from build123d import *

# Parameters (mm, degrees)
SKETCH1_W           = 15
SKETCH1_H           = 28.0162
SKETCH1_R           = 0.889
BOSS_EXTRUDE1_DEPTH = 3.175
SKETCH1_3_W         = 15
SKETCH1_3_H         = 12.7
SKETCH1_3_R         = 3.1115
BOSS_EXTRUDE2_DEPTH = 12.7


with BuildPart() as part:
    # Sketch1 → Boss-Extrude1 (new body)
    with BuildSketch(Plane(origin=(0, 0, 0), x_dir=(1, 0, 0), z_dir=(0, 1, 0))):
        with Locations((7.5, -26.7081)):
            Rectangle(SKETCH1_W, SKETCH1_H)
        with Locations(Location((3.69, -38.9262, 0), (0, 0, 270))):
            Circle(SKETCH1_R, mode=Mode.SUBTRACT)
        with Locations(Location((3.69, -31.3062, 0), (0, 0, 270))):
            Circle(SKETCH1_R, mode=Mode.SUBTRACT)
        with Locations(Location((11.31, -38.9262, 0), (0, 0, 270))):
            Circle(SKETCH1_R, mode=Mode.SUBTRACT)
        with Locations(Location((11.31, -31.3062, 0), (0, 0, 270))):
            Circle(SKETCH1_R, mode=Mode.SUBTRACT)
    extrude(amount=BOSS_EXTRUDE1_DEPTH)

    # Sketch1_3 → Boss-Extrude2 (add)
    with BuildSketch(Plane(origin=(0, 0, 0), x_dir=(1, 0, 0), z_dir=(0, 1, 0))):
        with Locations((7.5, -6.35)):
            Rectangle(SKETCH1_3_W, SKETCH1_3_H)
        with Locations(Location((7.5, -5.6515, 0), (0, 0, 270))):
            Circle(SKETCH1_3_R, mode=Mode.SUBTRACT)
    extrude(amount=BOSS_EXTRUDE2_DEPTH)


solid = part.part
Verification items for the finished model (mm, model axes). A direction names the side the tool comes from. Coordinates: 2 decimals unless noted, no trailing zeros. Write each loop counter-clockwise with the first axis right and the second up, starting at its lowest first coordinate (ties: lowest second). Pieces come first, ordered by that corner, then holes. Notation, with made-up numbers: (24, -15) -> (35, -15) arc R12 ccw to (35, -8) -> close; hole circle Ø1 at (47, 61.5). An arc over 180 degrees is marked (long way). One line per item, written item: value. Start each with the question number.
Q1. Thickness scan on L1, parallel to Z at x = 13, y = 10.25; L2, parallel to Y at x = 2.25, z = 35.5 (3 decimals); L3, parallel to X at y = 11, z = 5. Record the ranges inside material, lowest first. Write a range as from..to.
Q2. Access from +Z, -Z, +X, -X, +Y, -Y to the whole of each face (thin tool, end or side, straight path). Record for faces 4 (the flat face through (7, 3.175, 27)), 5 (the flat face through (7, 6, 0)).
Q3. Cross-section at A-A on x = 7.5. Enter the section's corners in (y, z) (3 decimals).
Q4. Cross-section at C-C on y = 2.5. Enter the section's corners in (x, z).
Q5. Cross-section at B-B on x = 11.31. Enter the section's corners in (y, z) (3 decimals).
Q6. Go/stop test with flat-tipped pins: P1, Ø5, axis at x = 2.5, y = 9, coming from the +Z side; P2, Ø4, axis at x = 2.5, y = 5, coming from the +Z side; P3, Ø4.5, axis at x = 10.5, z = 30, coming from the +Y side (3 decimals). Record where each tip stops, or that it passes through.
Q7. Cross-section at D-D on z = 31.5. Enter the section's corners in (x, y) (3 decimals).
Q8. Mould release check, pull along X, two halves, no side actions. Record for faces 1 (the cylindrical face through (3.73, 1.57, 30.42)), 2 (the flat face through (7, 8, 12.7)), 3 (the flat face through (0, 5, 12)): pulls with the +X half, pulls with the -X half, needs draft (parallel to the pull), parting line crosses it, or undercut.
Checked values:
1. L1: z = 0..12.7
1. L2: y = 0..3.175
1. L3: x = 0..4.46, 10.54..15
2. face 4: +Z, +X, -X, +Y
2. face 5: -Z, +X, -X, +Y, -Y
3. outline: (0, 0) -> (12.7, 0) -> (12.7, 2.54) -> (0, 2.54) -> close; (0, 8.763) -> (12.7, 8.763) -> (12.7, 12.7) -> (3.175, 12.7) -> (3.175, 40.716) -> (0, 40.716) -> close
4. outline: (0, 0) -> (15, 0) -> (15, 40.72) -> (0, 40.72) -> close; hole circle Ø1.78 at (3.69, 31.31); hole circle Ø1.78 at (3.69, 38.93); hole circle Ø6.22 at (7.5, 5.65); hole circle Ø1.78 at (11.31, 31.31); hole circle Ø1.78 at (11.31, 38.93)
5. outline: (0, 0) -> (12.7, 0) -> (12.7, 12.7) -> (3.175, 12.7) -> (3.175, 30.417) -> (0, 30.417) -> close; (0, 32.195) -> (3.175, 32.195) -> (3.175, 38.037) -> (0, 38.037) -> close; (0, 39.815) -> (3.175, 39.815) -> (3.175, 40.716) -> (0, 40.716) -> close
6. P1: stops at z = 12.7
6. P2: stops at z = 40.72
6. P3: stops at y = 3.175
7. outline: (0, 0) -> (2.822, 0) -> (2.822, 3.175) -> (0, 3.175) -> close; (4.558, 0) -> (10.442, 0) -> (10.442, 3.175) -> (4.558, 3.175) -> close; (12.178, 0) -> (15, 0) -> (15, 3.175) -> (12.178, 3.175) -> close
8. face 1: undercut
8. face 2: needs draft
8. face 3: pulls with the -X half
